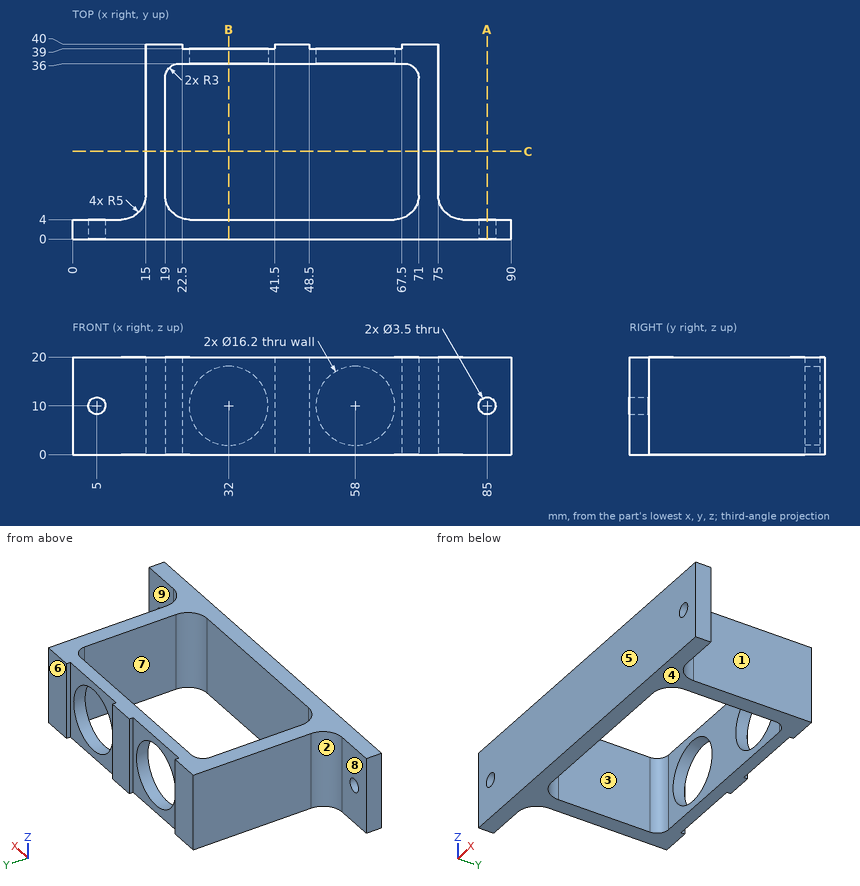
For this review, use the dimensioned drawing (mm, ordinates from the lowest corner) and the shaded views. A direction names the side the tool comes from. Coordinates: 2 decimals unless noted, no trailing zeros. Loops run counter-clockwise (first coordinate to the right, second up) from the corner with the lowest first, then second, coordinate; pieces in that order, holes last. Notation, with made-up numbers: (-17.75, 43.25) - (-8.75, 43.25) arc R23 cw to (-8.75, 71.25) - close; hole circle Ø10 at (-17, 76). An arc over 180 degrees is marked (long way). Use one line per item in the form item = value. Start each with the question number.
1) For the marked faces 5, 6, 7, 8 and 9, list the 3-axis set-ups (+Z, -Z, +X, -X, +Y, -Y) from which the entire face can be reached by the end or side of a thin tool; tool diameter is ignored.
2) For pin 1 (4 mm diameter, centred on x = 71, z = 16.5, fed in from -Y); pin 2 (12 mm diameter, centred on y = 19.5, z = 12.5, fed in from -X); pin 3 (1.1 mm diameter, centred on y = 39.5, z = 13.5, fed in from +X); pin 4 (10 mm diameter, centred on y = 9.5, z = 3, fed in from -X), all flat-tipped, find the tip position at first contact; note any pin that passes through.
3) To check wall thickness, follow probe 1 along X at (y, z) = (1.45, 10); probe 2 along X at (y, z) = (38, 10); probe 3 along X at (y, z) = (9.5, 5.5). State the ranges of each line that lie inside material, in increasing order. Write a range as from..to.
4) Draft analysis for pull direction X (two halves, no side actions). For the marked faces 1, 2, 3 and 4, state which applies: released by +X, released by -X, zero draft, split by the parting line, or undercut.
5) Take a section at C-C (y = 18). State the section outline as (x, z) points, plus the area to 3 significant figures.
6) Take a section at B-B (x = 32). State the section outline as (y, z) points.
7) Take a section at A-A (x = 85). State the section outline as (y, z) points.
From the geometry:
q1.face_5 = +Z, -Z, +X, -X, -Y
q1.face_6 = +Z, -Z, +X, -X, +Y
q1.face_7 = +Z, -Z
q1.face_8 = +Z, -Z, -X, +Y
q1.face_9 = +Z, -Z, +X, +Y
q2.pin_1 = 0
q2.pin_2 = 15
q2.pin_3 = 75
q2.pin_4 = 12.18
q3.probe_1 = 0..3.25, 6.75..83.25, 86.75..90
q3.probe_2 = 15..23.9, 40.1..49.9, 66.1..75
q3.probe_3 = 15..19, 71..75
q4.face_1 = released by +X
q4.face_2 = released by -X
q4.face_3 = undercut
q4.face_4 = zero draft
q5.outline = (15, 0) - (19, 0) - (19, 20) - (15, 20) - close; (71, 0) - (75, 0) - (75, 20) - (71, 20) - close
q5.area = 160 mm2
q6.outline = (0, 0) - (4, 0) - (4, 20) - (0, 20) - close; (36, 0) - (39, 0) - (39, 1.9) - (36, 1.9) - close; (36, 18.1) - (39, 18.1) - (39, 20) - (36, 20) - close
q7.outline = (0, 0) - (4, 0) - (4, 8.25) - (0, 8.25) - close; (0, 11.75) - (4, 11.75) - (4, 20) - (0, 20) - close
